```python
from build123d import *

# Parameters (mm, degrees)
BOSS_EXTRUDE1_DEPTH = 0.2
BOSS_EXTRUDE2_DEPTH = 12.58
SKETCH1_4_W         = 162.49
SKETCH1_4_H         = 2
BOSS_EXTRUDE3_DEPTH = 15.58


# Read off the part's stored shape, not the designer's step: Boss-Extrude2
with BuildPart() as part:
    # Sketch1 → Boss-Extrude1 (new body)
    with BuildSketch(Plane(origin=(0, 0, 0), x_dir=(1, 0, 0), z_dir=(0, 1, 0))):
        Polygon((-115, 0), (-111, -6.92820323), (111, -6.92820323), (115, 0), (15.625, 172.122549002), (13.892949192, 171.122549002), (2.845299462, 190.25763964), (-2.845299462, 190.25763964), (-13.892949192, 171.122549002), (-15.625, 172.122549002), align=None)
    extrude(amount=BOSS_EXTRUDE1_DEPTH)

    # Boss-Extrude2 outline → Boss-Extrude2 (add)
    with BuildSketch(Plane(origin=(0, 0, 0), x_dir=(1, 0, 0), z_dir=(0, 1, 0))):
        Polygon((15.625, 172.122549002), (4, 192.25763964), (-4, 192.25763964), (-15.625, 172.122549002), (-13.892949192, 171.122549002), (-2.845299462, 190.25763964), (2.845299462, 190.25763964), (13.892949192, 171.122549002), align=None)
        Polygon((62, 91.798692801), (57, 100.458946839), (55.267949192, 99.458946839), (60.267949192, 90.798692801), align=None)
        Polygon((-95.137949192, 30.402081141), (-96.87, 31.402081141), (-115, 0), (-111, -6.92820323), (-74.74, -6.92820323), (-74.74, -4.92820323), (-109.845299462, -4.92820323), (-112.690598923, 0), align=None)
        Polygon((115, 0), (103.375, 20.135090638), (101.642949192, 19.135090638), (112.690598923, 0), (109.845299462, -4.92820323), (87.75, -4.92820323), (87.75, -6.92820323), (111, -6.92820323), align=None)
    extrude(amount=BOSS_EXTRUDE2_DEPTH)

    # Sketch1<4> → Boss-Extrude3 (add)
    with BuildSketch(Plane(origin=(0, 0, 0), x_dir=(1, 0, 0), z_dir=(0, 1, 0))):
        Polygon((-15.625, 172.122549002), (-96.87, 31.402081141), (-95.137949192, 30.402081141), (-13.892949192, 171.122549002), align=None)
        with Locations((6.505, -5.92820323)):
            Rectangle(SKETCH1_4_W, SKETCH1_4_H)
        Polygon((57, 100.458946839), (15.625, 172.122549002), (13.892949192, 171.122549002), (55.267949192, 99.458946839), align=None)
        Polygon((101.642949192, 19.135090638), (103.375, 20.135090638), (62, 91.798692801), (60.267949192, 90.798692801), align=None)
    extrude(amount=BOSS_EXTRUDE3_DEPTH)


solid = part.part
```
Input: part model. Units: mm. Frame: model coordinates. A direction names the side the tool comes from. Give positions to 0.01 mm unless a question says otherwise; leave off trailing zeros. Loops run counter-clockwise (first coordinate to the right, second up) from the corner with the lowest first, then second, coordinate; pieces in that order, holes last.
1) Reachability of faces 4 (the flat face through (112.972, 6.202, 3.513)), 5 (the flat face through (-108.4, 12.58, -8.1)), 6 (the flat face through (110, 12.58, -5)), 7 (the flat face through (35, 15.58, -136)), 8 (the flat face through (-111.248, 6.303, 2.499)) from +Z, -Z, +X, -X, +Y, -Y: full face, straight path, thin tool, end or side. Return the list, or none.
A:
face 4: +Z, +X, +Y, -Y
face 5: +Z, -X, +Y
face 6: +Z, +X, +Y
face 7: +Z, -Z, +X, -X, +Y
face 8: +Y
2) Line query: L1, parallel to Y at x = 104, z = -12.5; L2, parallel to Z at x = 14, y = 6; L3, parallel to Z at x = -77, y = 10.25. Output: solid intervals per line, ascending.
A:
L1: y = 0 to 0.2
L2: z = -174.94 to -170.94, 4.93 to 6.93
L3: z = -65.82 to -61.82, 4.93 to 6.93
3) Section query D-D on x = -59.5. Return the cut outline in (y, z).
A:
outline: (0, -96.13) - (15.58, -96.13) - (15.58, -92.13) - (0.2, -92.13) - (0.2, 4.93) - (15.58, 4.93) - (15.58, 6.93) - (0, 6.93) - close
4) Section query A-A on y = 5.25. Return the cut outline in (x, z) (3 decimals).
A:
outline: (-115, 0) - (-4, -192.258) - (4, -192.258) - (115, 0) - (111, 6.928) - (-111, 6.928) - close; hole (-112.691, 0) - (-2.845, -190.258) - (2.845, -190.258) - (112.691, 0) - (109.845, 4.928) - (-109.845, 4.928) - close
5) Mould query, pull axis Z, two halves, no side actions, for faces 1 (the flat face through (-113.028, 6.202, 3.416)), 2 (the flat face through (-2, 0.2, -72)), 3 (the flat face through (-2, 0, -72)). Classes: released by +Z, released by -Z, zero draft, split by the parting line, or undercut.
A:
face 1: released by +Z
face 2: undercut
face 3: zero draft
6) Section query C-C on x = 47. Return the cut outline in (y, z).
A:
outline: (0, -117.78) - (15.58, -117.78) - (15.58, -113.78) - (0.2, -113.78) - (0.2, 4.93) - (15.58, 4.93) - (15.58, 6.93) - (0, 6.93) - close
7) Contact query for flat-ended pins moving along their axis: pin 1 (0.6 mm diameter, centred on y = 14.5, z = 6, fed in from -X); pin 2 (3.5 mm diameter, centred on x = 59, z = -96, fed in from +Y); pin 3 (8 mm diameter, centred on y = 6.5, z = -19, fed in from -X). Output: stop coordinate, or through.
A:
pin 1: stops at x = -74.74
pin 2: stops at y = 12.58
pin 3: stops at x = -106.34
8) Section query B-B on z = -108.5. Return the cut outline in (x, y).
A:
outline: (-52.36, 0) - (52.36, 0) - (52.36, 15.58) - (50.05, 15.58) - (50.05, 0.2) - (-50.05, 0.2) - (-50.05, 15.58) - (-52.36, 15.58) - close
